Work out the finished part from the listing and answer in its coordinate system (mm). A direction names the side the tool comes from. Coordinates: 2 decimals unless noted, no trailing zeros. Loops run counter-clockwise (first coordinate to the right, second up) from the corner with the lowest first, then second, coordinate; pieces in that order, holes last.
```python
from build123d import *

# Parameters (mm, degrees)
SKETCH_1_R          = 13.75
EXTRUDE_1_DEPTH     = 24
SKETCH_2_R          = 4.45
EXTRUDE_2_DEPTH     = 2
SKETCH_3_R          = 1
CUT_EXTRUDE_1_DEPTH = 6


with BuildPart() as part:
    # 草图1 → 凸台-拉伸1 (new body)
    with BuildSketch(Plane.XY):
        Circle(SKETCH_1_R)
    extrude(amount=EXTRUDE_1_DEPTH)

    # 草图2 → 凸台-拉伸2 (add)
    with BuildSketch(Plane.XY.offset(24)):
        Circle(SKETCH_2_R)
    extrude(amount=EXTRUDE_2_DEPTH)

    # 草图3 → 切除-拉伸1 (cut)
    with BuildSketch(Plane.XY.offset(26)):
        with Locations((6, 0)):
            Circle(SKETCH_3_R)
        with Locations((-3, -5.196152423)):
            Circle(SKETCH_3_R)
        with Locations((-3, 5.196152423)):
            Circle(SKETCH_3_R)
    extrude(amount=-CUT_EXTRUDE_1_DEPTH, mode=Mode.SUBTRACT)


solid = part.part
```
1. A cutting plane is placed at C-C, the plane z = 12.25. Give the vertices of the cut face in (x, y).
2. Determine the mould class of faces 3 (the flat face through (0, 0, 26)), 4 (the cylindrical face through (-3.13, 6.188, 22.028)), 5 (the cylindrical face through (-0.965, -4.344, 24.986)) for opening direction Y: released by +Y, released by -Y, zero draft, split by the parting line, or undercut.
3. For faces 1 (the cylindrical face through (-2.981, -13.423, 11.832)), 2 (the flat face through (0, -6, 24)), determine the directions among +Z, -Z, +X, -X, +Y, -Y from which every point of the face is accessible in a straight line to the end or side of a thin tool.
4. Straight lines are drawn through the part: probe 1 along Y at (x, z) = (-3, 22.65); probe 2 along Z at (x, y) = (8.5, 9.5); probe 3 along Y at (x, z) = (-7.75, 13). For each, find the intervals that lie inside material, in ascending order.
5. A cutting plane is placed at D-D, the plane x = -3. Give the vertices of the cut face in (y, z).
6. A cutting plane is placed at A-A, the plane y = 0. Give the vertices of the cut face in (x, z), then the cut area to 3 significant figures.
7. Each of these flat-tipped pins is pushed along its axis until it touches: P1, Ø1.5, axis at x = 8, z = 23, coming from the +Y side; P2, Ø3, axis at x = 10.5, y = 11, coming from the +Z side; P3, Ø8, axis at x = -7, z = 5, coming from the -Y side. Where does it stop, or does it pass through?
8. A cutting plane is placed at B-B, the plane x = 0. Give the vertices of the cut face in (y, z), then the cut area to 3 significant figures.
Answers below:
1. outline: circle Ø27.5 at (0, 0)
2. face 3: zero draft
2. face 4: undercut
2. face 5: split by the parting line
3. face 1: +Z, -Z
3. face 2: +Z
4. probe 1: y = -13.42 to -6.2, -4.2 to 4.2, 6.2 to 13.42
4. probe 2: z = 0 to 24
4. probe 3: y = -11.36 to 11.36
5. outline: (-13.42, 0) - (13.42, 0) - (13.42, 24) - (6.2, 24) - (6.2, 20) - (4.2, 20) - (4.2, 24) - (3.29, 24) - (3.29, 26) - (-3.29, 26) - (-3.29, 24) - (-4.2, 24) - (-4.2, 20) - (-6.2, 20) - (-6.2, 24) - (-13.42, 24) - close
6. outline: (-13.75, 0) - (13.75, 0) - (13.75, 24) - (7, 24) - (7, 20) - (5, 20) - (5, 24) - (4.45, 24) - (4.45, 26) - (-4.45, 26) - (-4.45, 24) - (-13.75, 24) - close
6. area: 670 mm2
7. P1: stops at y = 11.68
7. P2: stops at z = 24
7. P3: stops at y = -13.42
8. outline: (-13.75, 0) - (13.75, 0) - (13.75, 24) - (4.45, 24) - (4.45, 26) - (-4.45, 26) - (-4.45, 24) - (-13.75, 24) - close
8. area: 678 mm2
